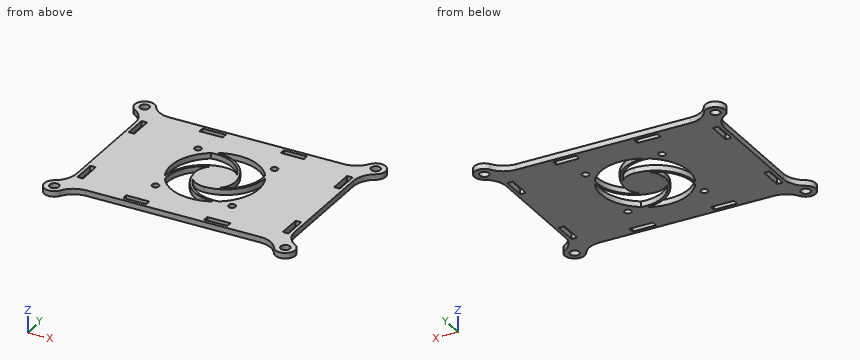
```python
from build123d import *

# Parameters (mm, degrees)
F0_R     = 2
F0_W     = 2.4
F0_H     = 10
F0_W_2   = 10
F0_H_2   = 2.4
F0_R_2   = 1.5
F1_DEPTH = 2.4


with BuildPart() as f1:
    # F0 (on Top) → F1 (new body)
    with BuildSketch(Plane.XY):
        with BuildLine():
            ThreePointArc((46.111466, 37.36014), (42.463054, 33.799465), (37.533481, 32.5))
            Line((37.533481, 32.5), (-37.533481, 32.5))
            ThreePointArc((-37.533481, 32.5), (-42.463054, 33.799465), (-46.111466, 37.36014))
            ThreePointArc((-46.111466, 37.36014), (-52.859026, 38.171979), (-51.965035, 31.434812))
            ThreePointArc((-51.965035, 31.434812), (-48.329658, 27.777326), (-47, 22.794839))
            Line((-47, 22.794839), (-47, 0))
            Line((-47, 0), (-47, -22.794839))
            ThreePointArc((-47, -22.794839), (-48.329658, -27.777326), (-51.965035, -31.434812))
            ThreePointArc((-51.965035, -31.434812), (-52.859026, -38.171979), (-46.111466, -37.36014))
            ThreePointArc((-46.111466, -37.36014), (-42.463054, -33.799465), (-37.533481, -32.5))
            Line((-37.533481, -32.5), (37.533481, -32.5))
            ThreePointArc((37.533481, -32.5), (42.463054, -33.799465), (46.111466, -37.36014))
            ThreePointArc((46.111466, -37.36014), (52.859026, -38.171979), (51.965035, -31.434812))
            ThreePointArc((51.965035, -31.434812), (48.329658, -27.777326), (47, -22.794839))
            Line((47, -22.794839), (47, 22.794839))
            ThreePointArc((47, 22.794839), (48.329658, 27.777326), (51.965035, 31.434812))
            ThreePointArc((51.965035, 31.434812), (52.859026, 38.171979), (46.111466, 37.36014))
        make_face()
        with Locations((-49.8, -35.15)):
            Circle(F0_R, mode=Mode.SUBTRACT)
        with Locations((-44.3, -20)):
            Rectangle(F0_W, F0_H, mode=Mode.SUBTRACT)
        with Locations((-17.5, -29.8)):
            Rectangle(F0_W_2, F0_H_2, mode=Mode.SUBTRACT)
        with Locations((-16.49, -16.5)):
            Circle(F0_R_2, mode=Mode.SUBTRACT)
        with BuildLine():
            ThreePointArc((-15.883599, -10.426471), (-13.617771, -0.10022), (-5.406647, 6.558824))
            ThreePointArc((-5.406647, 6.558824), (-7.687864, 3.625845), (-8.5, 0))
            ThreePointArc((-8.5, 0), (-3.526013, -12.015615), (8.485294, -16.999994))
            ThreePointArc((8.485294, -16.999994), (-4.948387, -18.344303), (-15.883599, -10.426471))
        make_face(mode=Mode.SUBTRACT)
        with Locations((17.5, -29.8)):
            Rectangle(F0_W_2, F0_H_2, mode=Mode.SUBTRACT)
        with Locations((49.8, -35.15)):
            Circle(F0_R, mode=Mode.SUBTRACT)
        with Locations((44.3, -20)):
            Rectangle(F0_W, F0_H, mode=Mode.SUBTRACT)
        with Locations((16.51, -16.5)):
            Circle(F0_R_2, mode=Mode.SUBTRACT)
        with BuildLine():
            ThreePointArc((-6.558824, -5.406647), (-3.625845, -7.687864), (0, -8.5))
            ThreePointArc((0, -8.5), (12.015615, -3.526013), (16.999994, 8.485294))
            ThreePointArc((16.999994, 8.485294), (18.344303, -4.948387), (10.426471, -15.883599))
            ThreePointArc((10.426471, -15.883599), (0.10022, -13.617771), (-6.558824, -5.406647))
        make_face(mode=Mode.SUBTRACT)
        with BuildLine():
            ThreePointArc((-10.426471, 15.883599), (-0.10022, 13.617771), (6.558824, 5.406647))
            ThreePointArc((6.558824, 5.406647), (3.625845, 7.687864), (0, 8.5))
            ThreePointArc((0, 8.5), (-12.015615, 3.526013), (-16.999994, -8.485294))
            ThreePointArc((-16.999994, -8.485294), (-18.344303, 4.948387), (-10.426471, 15.883599))
        make_face(mode=Mode.SUBTRACT)
        with Locations((-16.49, 16.5)):
            Circle(F0_R_2, mode=Mode.SUBTRACT)
        with Locations((-44.3, 20)):
            Rectangle(F0_W, F0_H, mode=Mode.SUBTRACT)
        with Locations((-49.8, 35.15)):
            Circle(F0_R, mode=Mode.SUBTRACT)
        with Locations((-17.5, 29.8)):
            Rectangle(F0_W_2, F0_H_2, mode=Mode.SUBTRACT)
        with BuildLine():
            ThreePointArc((-8.485294, 16.999994), (4.948387, 18.344303), (15.883599, 10.426471))
            ThreePointArc((15.883599, 10.426471), (13.617771, 0.10022), (5.406647, -6.558824))
            ThreePointArc((5.406647, -6.558824), (7.687864, -3.625845), (8.5, 0))
            ThreePointArc((8.5, 0), (3.526013, 12.015615), (-8.485294, 16.999994))
        make_face(mode=Mode.SUBTRACT)
        with Locations((16.51, 16.5)):
            Circle(F0_R_2, mode=Mode.SUBTRACT)
        with Locations((17.5, 29.8)):
            Rectangle(F0_W_2, F0_H_2, mode=Mode.SUBTRACT)
        with Locations((44.3, 20)):
            Rectangle(F0_W, F0_H, mode=Mode.SUBTRACT)
        with Locations((49.8, 35.15)):
            Circle(F0_R, mode=Mode.SUBTRACT)
    extrude(amount=F1_DEPTH)


solid = f1.part
```
Here's how the part is built. I have some questions about the finished solid (model axes, mm). Round coordinates to 2 decimals unless told otherwise and drop trailing zeros. Loops run counter-clockwise (first coordinate to the right, second up) from the corner with the lowest first, then second, coordinate; pieces in that order, holes last. Notation, with made-up numbers: (-6.75, -21) -> (39.25, -21) arc R13 ccw to (39.25, -14) -> close; hole circle Ø6 at (6.5, 40.5). An arc over 180 degrees is marked (long way). Answer as CSV lines item,"result".
1. If we section it at C-C on y = -12: Please give me the cut outline in (x, z), plus the area to 3 significant figures.
Final values:
outline,"(-47, 0) -> (-14.73, 0) -> (-14.73, 2.4) -> (-47, 2.4) -> close; (-3.54, 0) -> (-2.08, 0) -> (-2.08, 2.4) -> (-3.54, 2.4) -> close; (14.73, 0) -> (47, 0) -> (47, 2.4) -> (14.73, 2.4) -> close"
area,"158 mm^2"
2. If we section it at B-B on x = 49.8: Please give me the cut outline in (y, z), plus the area to 3 significant figures.
Final values:
outline,"(-39.45, 0) -> (-37.15, 0) -> (-37.15, 2.4) -> (-39.45, 2.4) -> close; (-33.15, 0) -> (-29.73, 0) -> (-29.73, 2.4) -> (-33.15, 2.4) -> close; (29.73, 0) -> (33.15, 0) -> (33.15, 2.4) -> (29.73, 2.4) -> close; (37.15, 0) -> (39.45, 0) -> (39.45, 2.4) -> (37.15, 2.4) -> close"
area,"27.4 mm^2"
3. For pin 1 (0.7 mm diameter, centred on x = -44.5, z = 0.5, fed in from +Y); pin 2 (1.2 mm diameter, centred on y = 30, z = 1.5, fed in from -X); pin 3 (0.7 mm diameter, centred on y = 9.5, z = 1, fed in from -X), each with a flat end and sliding along its axis, tell me the tip position at first contact or that it passes through.
Final values:
pin 1,"stops at y = 35.68"
pin 2,"stops at x = -50.75"
pin 3,"stops at x = -47"
4. If I drill on L1, parallel to X at y = -20.5, z = 2.15; L2, parallel to Y at x = 49.8, z = 1.1; L3, parallel to X at y = -30.5, z = 0.2, over which ranges is the centre line in solid material (lowest first)?
Final values:
L1,"x = -47 to -45.5, -43.1 to 43.1, 45.5 to 47"
L2,"y = -39.45 to -37.15, -33.15 to -29.73, 29.73 to 33.15, 37.15 to 39.45"
L3,"x = -50.63 to -22.5, -12.5 to 12.5, 22.5 to 50.63"
5. If we section it at D-D on z = 1.6: Count the separate pieces of the cut face and the enclosed holes in it, plus the area to 3 significant figures.
Final values:
separate pieces,"1"
enclosed holes,"20"
area,"5,340 mm^2"
6. If we section it at A-A on y = 35.15: Please give me the cut outline in (x, z).
Final values:
outline,"(-54.1, 0) -> (-51.8, 0) -> (-51.8, 2.4) -> (-54.1, 2.4) -> close; (-47.8, 0) -> (-44.31, 0) -> (-44.31, 2.4) -> (-47.8, 2.4) -> close; (44.31, 0) -> (47.8, 0) -> (47.8, 2.4) -> (44.31, 2.4) -> close; (51.8, 0) -> (54.1, 0) -> (54.1, 2.4) -> (51.8, 2.4) -> close"
